CAD build for the part. Positions are in the model's coordinates, mm. Coordinates: 2 decimals unless noted, no trailing zeros. Order: outer loops, then holes, each group sorted by start corner. A loop starts at its lowest first (then second) coordinate and runs counter-clockwise, first axis right, second up. Notation, with made-up numbers: (9.25, -2) - (28.25, -2) arc R11 ccw to (28.25, 15) - close; hole circle Ø2 at (81.5, 4.25). An arc over 180 degrees is marked (long way). Use one line per item in the form item = value.
Autodesk Fusion 360 part; units mm, degrees
sketch "Sketch1" plane through (0, 0, 0) normal (0, 0, 1) x (1, 0, 0)
  circle A0 centre (-13.6792, 145.0658) radius 1.5
  circle A1 centre (165.3208, 145.0658) radius 1.5
  circle A2 centre (-13.6792, 12.1658) radius 1.5
  circle A3 centre (165.3208, 12.1658) radius 1.5
  circle A4 centre (43.3208, 42.5182) radius 1.5
  circle A5 centre (108.3208, 41.4658) radius 1.5
  circle A6 centre (43.3208, 116.7382) radius 1.5
  circle A7 centre (108.3208, 115.7658) radius 1.5
  line L0 (-23.5792, 156.1658) -> (175.3708, 156.1658)
  line L1 (175.3708, 156.1658) -> (175.3708, 1.0658)
  line L2 (175.3708, 1.0658) -> (-23.5792, 1.0658)
  line L3 (-23.5792, 1.0658) -> (-23.5792, 156.1658)
  circle A8 centre (21.2, 108.6782) radius 1.25
  circle A9 centre (70, 108.6782) radius 1.25
  circle A10 centre (21.2, 50.5782) radius 1.25
  circle A11 centre (70, 50.5782) radius 1.25
  circle A12 centre (95, 97.3658) radius 1.25
  circle A13 centre (131.3, 97.3658) radius 1.25
  circle A14 centre (95, 59.8658) radius 1.25
  circle A15 centre (131.3, 59.8658) radius 1.25
  line L4 (-10.8, 97.1908) -> (1.2, 97.1908)
  line L5 (1.2, 97.1908) -> (1.2, 60.0408)
  line L6 (1.2, 60.0408) -> (-10.8, 60.0408)
  line L7 (-10.8, 60.0408) -> (-10.8, 97.1908)
  line L8 (151.3, 97.1908) -> (163.3, 97.1908)
  line L9 (151.3, 60.0408) -> (151.3, 97.1908)
  line L10 (163.3, 60.0408) -> (151.3, 60.0408)
  line L11 (163.3, 97.1908) -> (163.3, 60.0408)
  dimension "d1" = 3
  dimension "d2" = 3
  dimension "d3" = 3
  dimension "d4" = 3
  dimension "d14" = 3
  dimension "d15" = 3
  dimension "d16" = 3
  dimension "d17" = 3
  dimension "d21" = 74.3
  dimension "d33" = 67.05
  dimension "d34" = 67.05
  dimension "d36" = 65
  dimension "d37" = 66.9
  dimension "d38" = 65
  dimension "d39" = 11.1
  dimension "d40" = 9.9
  dimension "d41" = 11.1
  dimension "d42" = 10.05
  dimension "d43" = 10.05
  dimension "d44" = 11.1
  dimension "d45" = 11.1
  dimension "d46" = 9.9
  dimension "d47" = 40.4
  dimension "d48" = 40.4
  dimension "d49" = 2.5
  dimension "d50" = 2.5
  dimension "d51" = 2.5
  dimension "d52" = 2.5
  dimension "d53" = 58.1
  dimension "d54" = 58.1
  dimension "d55" = 48.8
  dimension "d56" = 48.8
  dimension "d65" = 2.5
  dimension "d66" = 2.5
  dimension "d67" = 2.5
  dimension "d68" = 2.5
  dimension "d71" = 36.3
  dimension "d72" = 36.3
  dimension "d73" = 37.5
  dimension "d74" = 37.5
  dimension "d79" = 18.4
  dimension "d80" = 37.15
  dimension "d81" = 12
  dimension "d82" = 37.15
  dimension "d83" = 12
  dimension "d84" = 8.06
  dimension "d85" = 8.06
  dimension "d86" = 18.4
  dimension "d88" = 25
  dimension "d91" = 20
  dimension "d92" = 47.875
  dimension "d93" = 20
  dimension "d94" = 47.875
extrude "Extrude1" add sketch "Sketch1" along normal blind 3.5
Item 1: Cut at A-A, the plane y = 88. Write the cut outline in (x, z).
Derived:
outline = (-23.58, 0) - (-10.8, 0) - (-10.8, 3.5) - (-23.58, 3.5) - close; (1.2, 0) - (151.3, 0) - (151.3, 3.5) - (1.2, 3.5) - close; (163.3, 0) - (175.37, 0) - (175.37, 3.5) - (163.3, 3.5) - close
Item 2: Cut at B-B, the plane z = 2.3. State how many separate pieces and enclosed holes the cut face has, plus the area to 3 significant figures.
Derived:
separate_pieces = 1
enclosed_holes = 18
area = 29,900 mm²
Item 3: Drill centre lines: line 1 (Y direction, x = 21.2, z = 2.4); line 2 (X direction, y = 67, z = 1.45); line 3 (Y direction, x = 21.5, z = 1.85). Where is each one in solid material? Low to high. Write a range as [from, to].
Derived:
line_1 = [1.07, 49.33], [51.83, 107.43], [109.93, 156.17]
line_2 = [-23.58, -10.8], [1.2, 151.3], [163.3, 175.37]
line_3 = [1.07, 49.36], [51.79, 107.46], [109.89, 156.17]
